Read the model definition and answer for the solid it produces. Units are mm, in the model's axes. A direction names the side the tool comes from. Coordinates: 2 decimals unless noted, no trailing zeros. Write each loop counter-clockwise with the first axis right and the second up, starting at its lowest first coordinate (ties: lowest second). Pieces come first, ordered by that corner, then holes.
Item 1: Determine the mould class of faces 5 (the face through (528.986, 0.676, 154.297)), 6 (the face through (-11, 1, 0)), 7 (the face through (549.297, -0.753, 173.986)) for opening direction X: released by +X, released by -X, zero draft, split by the parting line, or undercut.
Item 2: Section B-B (x = 508) is taken. Give the vertices of the cut face in (y, z).
Item 3: Straight lines are drawn through the part: probe 1 along Y at (x, z) = (379.5, 128); probe 2 along Z at (x, y) = (165.5, -16.5); probe 3 along X at (y, z) = (39.5, 88.5). For each, find the intervals that lie inside material, in ascending order.
Item 4: A tool of negligible diameter and unlimited length cuts with its end or side. For faces 1 (the face through (475, -1, 120)), 2 (the face through (292, 1, 180)), 3 (the face through (292, -1, 60)), 4 (the face through (302, -51.067, 121)), from which of +Z, -Z, +X, -X, +Y, -Y can it reach the whole face along a straight path? Write none if from no direction.
Item 5: Each of these flat-tipped pins is pushed along its axis until it touches: P1, Ø4, axis at x = -4.5, z = 162, coming from the +Y side; P2, Ø12, axis at x = 257.5, y = -6, coming from the -Z side; P3, Ø1.5, axis at x = 395.5, y = 51, coming from the +Z side. Where does it stop, or does it pass through?
Item 6: Section D-D (x = 288.5) is taken. Give the vertices of the cut face in (y, z).
Item 7: Section C-C (z = 146.5) is taken. Give the vertices of the cut face in (x, y).
Item 8: Section A-A (y = 0) is taken. Give the vertices of the cut face in (x, z).
Autodesk Inventor part; units mm, degrees
ref_plane "YZ Plane" through (0, 0, 0) normal (1, 0, 0) x (0, 1, 0)
ref_plane "XZ Plane" through (0, 0, 0) normal (0, 1, 0) x (-1, 0, 0)
ref_plane "XY Plane" through (0, 0, 0) normal (0, 0, 1) x (1, 0, 0)
sketch "Sketch1" plane through (0, 0, 0) normal (0, 0, 1) x (1, 0, 0)
  circle A0 centre (0, 0) radius 75
  dimension "d0" = 150
extrude "Extrusion1" add sketch "Sketch1" along normal blind 240
sketch "Sketch2" plane through (0, 0, 240) normal (0, 0, 1) x (1, 0, 0)
  line L0 (95, -87.5905) -> (55, -87.5905)
  line L1 (55, -87.5905) -> (55, 87.5905)
  line L2 (55, 87.5905) -> (95, 87.5905)
  line L3 (95, 87.5905) -> (95, -87.5905)
  circle A0 centre (0, 0) radius 75
  line L4 (95, -87.5905) -> (55, 87.5905) construction
  line L5 (55, -87.5905) -> (95, 87.5905) construction
  point P0 (75, 0)
  point P1 (55, 50.9902)
  point P2 (55, -50.9902)
  dimension "d3" = 40
extrude "Extrusion2" cut sketch "Sketch2" against normal blind 240 contours L1 A0 picked at (65.2118, -7.3649)
sketch "Sketch3" plane through (55, -50.9902, 240) normal (1, 0, 0) x (0, 0, -1)
  line L0 (0, 101.9804) -> (240, 101.9804)
  line L1 (59.9997, -0.0764) -> (179.9997, -0.0764)
  line L2 (179.9997, -0.0764) -> (179.9997, 101.9804)
  line L3 (179.9997, 101.9804) -> (59.9997, 101.9804)
  line L4 (59.9997, 101.9804) -> (59.9997, -0.0764)
  line L5 (59.9997, -0.0764) -> (179.9997, 101.9804) construction
  line L6 (179.9997, -0.0764) -> (59.9997, 101.9804) construction
  point P0 (240, 50.9902)
  point P1 (119.9997, 50.952)
  point P2 (59.9997, 101.9804)
  dimension "d6" = 240
  dimension "d7" = 60
  dimension "d8" = 102.0568
extrude "Extrusion3" add sketch "Sketch3" along normal blind 500
sketch "Sketch4" plane through (55, 50.9902, 180.0003) normal (0, 1, 0) x (1, 0, 0)
  line L0 (420, 20) -> (480, 20)
  line L1 (480, 20) -> (480, 100)
  line L2 (480, 100) -> (420, 100)
  line L3 (420, 100) -> (420, 20)
  line L4 (420, 20) -> (480, 100) construction
  line L5 (480, 20) -> (420, 100) construction
  line L6 (0, 120) -> (500, 120)
  line L7 (500, 120) -> (500, 0)
  point P0 (-55, 180.0003)
  point P1 (450, 60)
  dimension "d11" = 80
  dimension "d12" = 40
  dimension "d13" = 60
  dimension "d14" = 20
  dimension "d15" = 60
extrude "Extrusion4" cut sketch "Sketch4" along normal mid plane 500
fillet "Fillet1" radius 20 2 edges at (555, -0.0382, 60.0003) (555, -0.0382, 180.0003)
fillet "Fillet2" radius 20 4 edges at (535, -0.0382, 160.0003) (535, -0.0382, 80.0003) (475, -0.0382, 160.0003) (475, -0.0382, 80.0003)
properties part number "Part2final"
Established:
1. face 5: undercut
1. face 6: zero draft
1. face 7: released by +X
2. outline: (-51.07, 60) - (50.99, 60) - (50.99, 80) - (-51.07, 80) - close; (-51.07, 160) - (50.99, 160) - (50.99, 180) - (-51.07, 180) - close
3. probe 1: y = -51.07 to 50.99
3. probe 2: z = 60 to 180
3. probe 3: x = -63.76 to 478.64, 531.36 to 555
4. face 1: +Y, -Y
4. face 2: +Z, +X, +Y, -Y
4. face 3: -Z, +X, +Y, -Y
4. face 4: +Z, -Z, +X, -Y
5. P1: stops at y = 74.96
5. P2: stops at z = 60
5. P3: stops at z = 180
6. outline: (-51.07, 60) - (50.99, 60) - (50.99, 180) - (-51.07, 180) - close
7. outline: (55, -51.07) - (476.09, -51.07) - (476.09, 50.99) - (55, 50.99) arc R75 ccw (long way) to (55, -50.99) - close; (533.91, -51.07) - (555, -51.07) - (555, 50.99) - (533.91, 50.99) - close
8. outline: (-75, 0) - (55, 0) - (55, 60) - (535, 60) arc R20 ccw to (555, 80) - (555, 160) arc R20 ccw to (535, 180) - (55, 180) - (55, 240) - (-75, 240) - close; hole (475, 100) arc R20 ccw to (495, 80) - (515, 80) arc R20 ccw to (535, 100) - (535, 140) arc R20 ccw to (515, 160) - (495, 160) arc R20 ccw to (475, 140) - close
